For this review, take the finished solid that the model builds, in its own axes (mm). Face numbers are marked on the shaded views. A direction names the side the tool comes from. Give positions to 0.01 mm unless a question says otherwise; leave off trailing zeros. Write each loop counter-clockwise with the first axis right and the second up, starting at its lowest first coordinate (ties: lowest second). Pieces come first, ordered by that corner, then holes. Notation, with made-up numbers: M 64.25,52.5 L 92.25,52.5 A20 cw 92.25,80.5 Z; hole C 9,60.5 d9. An arc over 180 degrees is marked long. One line per item, written item: value. Start each with the question number.
Item 1: To check wall thickness, follow probe 1 along X at (y, z) = (5, 6); probe 2 along Z at (x, y) = (-6.5, 4.75); probe 3 along Z at (x, y) = (-26.5, 8.5). State the ranges of each line that lie inside material, in increasing order.
Item 2: Consider section C-C, the plane x = -90.15. Write out the cut boundary in (y, z), and give its area (3 significant figures).
Item 3: Tool access review of the marked faces 1, 2 and 3: name each direction out of +Z, -Z, +X, -X, +Y, -Y from which nothing blocks a thin tool from reaching the whole face with its end or side.
Item 4: Consider section D-D, the plane x = -64.5. Write out the cut boundary in (y, z), and give its area (3 significant figures).
Item 5: Clearance check with flat-ended pins moving along their axes: pin 1 Ø12 at (x, z) = (-45, 25.5) entering from +Y; pin 2 Ø12 at (x, z) = (-90.15, 33.8) entering from -Y; pin 3 Ø4 at (x, y) = (-30.5, 1) entering from -Z; pin 4 Ø5 at (x, y) = (-62.5, 1) entering from +Z. State where each tip first meets the part, or that it passes through.
Item 6: Mouldability with a two-part tool opening along X and no side actions: class the marked faces 4, 5, 6 and 7 as released by +X, released by -X, zero draft, split by the parting line, or undercut.
Item 7: Consider section B-B, the plane z = 13. Write out the cut boundary in (x, y), and give its area (3 significant figures).
Item 8: Consider section A-A, the plane x = -16. Write out the cut boundary in (y, z), and give its area (3 significant figures).
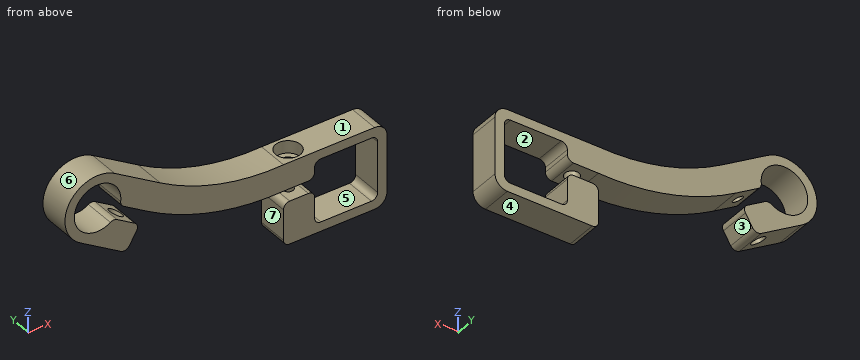
```python
from build123d import *

# Parameters (mm, degrees)
EXTRUDE_2_DEPTH             = 10
HOLE_WIZARD_M41_D           = 4.5
HOLE_WIZARD_M41_DEPTH       = 8.5
HOLE_WIZARD_M41_CBORE_D     = 8
HOLE_WIZARD_M41_CBORE_DEPTH = 4
HOLE_WIZARD_M41_2_REACH     = 112.256
HOLE_WIZARD_M41_2_BORE_R    = 2.25
FILLET_4_R                  = 4
FILLET_3_R                  = 2


with BuildPart() as part:
    # Эскиз1 → Бобышка-Вытянуть2 (new body)
    with BuildSketch(Plane(origin=(0, 0, 0), x_dir=(1, 0, 0), z_dir=(0, 1, 0))):
        with BuildLine():
            Line((3, 3), (-23.3, 3))
            Line((-23.3, 3), (-30.3, 3))
            Line((-30.3, 3), (-30.3, -10.8))
            Line((-30.3, -10.8), (-20.3, -10.8))
            Line((-20.3, -10.8), (-20.3, 0))
            Line((-20.3, 0), (0, 0))
            Line((0, 0), (0, -20.3))
            Line((0, -20.3), (-20.3, -20.3))
            Line((-20.3, -20.3), (-20.3, -14.8))
            Line((-20.3, -14.8), (-30.3, -14.8))
            ThreePointArc((-30.3, -14.8), (-53.235137158, -17.347468756), (-74.439305098, -26.452048677))
            Line((-74.439305098, -26.452048677), (-82.948576893, -31.704885388))
            ThreePointArc((-82.948576893, -31.704885388), (-96.531953846, -37.739627534), (-85.049711578, -28.30117667))
            Line((-85.049711578, -28.30117667), (-76.540439783, -23.048339959))
            Line((-76.540439783, -23.048339959), (-81.005350987, -15.815458933))
            Line((-81.005350987, -15.815458933), (-95.665478547, -24.865264615))
            ThreePointArc((-95.665478547, -24.865264615), (-99.084735385, -39.315478547), (-84.634521453, -42.734735385))
            Line((-84.634521453, -42.734735385), (-69.974393893, -33.684929703))
            ThreePointArc((-69.974393893, -33.684929703), (-50.914097819, -25.524407087), (-30.3, -23.3))
            Line((-30.3, -23.3), (-23.3, -23.3))
            Line((-23.3, -23.3), (3, -23.3))
            Line((3, -23.3), (3, 3))
        make_face()
    extrude(amount=EXTRUDE_2_DEPTH)

    # Эскиз4 → Отверстие обработанное метчиком M4x0.72 (revolve, cut)
    with BuildSketch(Plane(origin=(-25.3, 5, 10.8), x_dir=(0, -1, 0), z_dir=(1, 0, 0))):
        Polygon((0, 0), (0, 9.591420021), (1.65, 8.6), (1.65, 0), align=None)
    revolve(axis=Axis((-25.3, 5, 17.15), (0, 0, -1)), mode=Mode.SUBTRACT)

    # Эскиз6 → Отверстие обработанное метчиком M4x0.71 (revolve, cut)
    with BuildSketch(Plane(origin=(-78.693940996, 5, 29.078467033), x_dir=(-0.8509271795055905, 0, 0.5252836711517509), z_dir=(0, 1, 0))):
        Polygon((0, 0), (0, 8.491420021), (1.65, 7.5), (1.65, 0), align=None)
    revolve(axis=Axis((-82.029492307, 5, 23.675079443), (0.5252836711517508, 0, 0.8509271795055904)), mode=Mode.SUBTRACT)

    # Hole Wizard M41
    with Locations(Plane(origin=(-25.3, 5, 23.3), x_dir=(1, 0, 0), z_dir=(0, 0, 1))):
        with Locations((0, 0)):
            CounterBoreHole(HOLE_WIZARD_M41_D / 2, HOLE_WIZARD_M41_CBORE_D / 2, HOLE_WIZARD_M41_CBORE_DEPTH, depth=HOLE_WIZARD_M41_DEPTH)

    # Hole Wizard M41 2 bore → Hole Wizard M41 2 (cut, up to next)
    with BuildSketch(Plane(origin=(-15.282069591, 0, -24.756011063), x_dir=(-0.8509271795055892, 0, 0.525283671151753), z_dir=(-0.525283671151753, 0, -0.8509271795055892)), mode=Mode.PRIVATE) as hole_wizard_m41_2_sk1:
        with Locations((82.23725717, 5)):
            Circle(HOLE_WIZARD_M41_2_BORE_R)
    hole_wizard_m41_2_tool1 = extrude(hole_wizard_m41_2_sk1.sketch, amount=-HOLE_WIZARD_M41_2_REACH, mode=Mode.PRIVATE) & part.part
    add(hole_wizard_m41_2_tool1.solids().sort_by_distance((-85.259987, 5, 18.441877))[0], mode=Mode.SUBTRACT)

    # Скругление4
    fillet_4_edges = [part.edges().sort_by_distance(p)[0] for p in [
        (3, 5, -3),
        (3, 5, 23.3),
    ]]
    fillet(fillet_4_edges, radius=FILLET_4_R)

    # Скругление3
    fillet_3_edges = [part.edges().sort_by_distance(p)[0] for p in [
        (0, 5, 0),
        (-20.3, 5, 0),
        (-20.3, 5, 10.8),
        (-30.3, 5, 10.8),
        (-30.3, 5, -3),
        (-81.005350987, 5, 15.815458933),
        (-76.540439783, 5, 23.048339959),
        (-85.049711578, 5, 28.30117667),
        (-82.948576893, 5, 31.704885388),
        (-20.3, 5, 14.8),
        (-20.3, 5, 20.3),
        (0, 5, 20.3),
    ]]
    fillet(fillet_3_edges, radius=FILLET_3_R)


solid = part.part
```
Model answer:
1. probe 1: x = -30.3 to -26.95, -23.65 to -20.3, 0 to 3
1. probe 2: z = -3 to 0, 20.3 to 23.3
1. probe 3: z = -3 to 10.8, 14.8 to 19.3
2. outline: M 0,21.46 L 10,21.46 L 10,26.3 L 0,26.3 Z; M 0,41.3 L 10,41.3 L 10,44.3 L 0,44.3 Z
2. area: 78.4 mm2
3. face 1: +Z, +X, +Y, -Y
3. face 2: +Y, -Y
3. face 3: -Z, +Y, -Y
4. outline: M 0,21.26 L 10,21.26 L 10,30.63 L 0,30.63 Z
4. area: 93.8 mm2
5. pin 1: stops at y = 10
5. pin 2: passes through
5. pin 3: stops at z = -2.99
5. pin 4: stops at z = 30.89
6. face 4: zero draft
6. face 5: undercut
6. face 6: split by the parting line
6. face 7: released by -X
7. outline: M 0,0 L 3,0 L 3,10 L 0,10 Z
7. area: 30.0 mm2
8. outline: M 0,-3 L 10,-3 L 10,0 L 0,0 Z; M 0,20.3 L 10,20.3 L 10,23.3 L 0,23.3 Z
8. area: 60.0 mm2
